The model under review builds one solid part; all positions refer to its coordinate system, in mm. Coordinates: 2 decimals unless noted, no trailing zeros. Write each loop counter-clockwise with the first axis right and the second up, starting at its lowest first coordinate (ties: lowest second). Pieces come first, ordered by that corner, then holes.
1) Add section A-A, the plane z = -0.75. State the section outline as (x, y) points, then the cut area to 3 significant figures.
2) Mouldability with a two-part tool opening along Y and no side actions: class faces 1 (the flat face through (4, 0, 0.3)), 2 (the cylindrical face through (9.84, 15.43, -0.49)), 3 (the flat face through (-6, 0, 0.2)) as released by +Y, released by -Y, zero draft, split by the parting line, or undercut.
3) For P1, Ø10, axis at x = -14, y = -10.5, coming from the +Z side; P2, Ø11.5, axis at x = 5.5, y = -1.5, coming from the -Z side, all flat-tipped, find the tip position at first contact; note any pin that passes through.
4) For line 1 (Y direction, x = 0, z = -0.5); line 2 (Z direction, x = 11, y = -12.5); line 3 (X direction, y = -6.5, z = -0.15), list the stretches that pass through material, from the lowest coordinate up.
from build123d import *

# Parameters (mm, degrees)
SKETCH1_R           = 19.5
BOSS_EXTRUDE1_DEPTH = 0.3
SKETCH1_3_R         = 18.6
SKETCH1_3_R_2       = 18.3
BOSS_EXTRUDE2_DEPTH = 1
FILLET1_R           = 10
CUT_EXTRUDE1_START  = -0.1
CUT_EXTRUDE1_DEPTH  = 0.1


# Read off the part's stored shape, not the designer's step: Cut-Extrude1
with BuildPart() as part:
    # Sketch1 → Boss-Extrude1 (new body)
    with BuildSketch(Plane.XY):
        Circle(SKETCH1_R)
    extrude(amount=BOSS_EXTRUDE1_DEPTH)

    # Sketch1<3> → Boss-Extrude2 (add)
    with BuildSketch(Plane.XY):
        Circle(SKETCH1_3_R)
        Circle(SKETCH1_3_R_2, mode=Mode.SUBTRACT)
    extrude(amount=-BOSS_EXTRUDE2_DEPTH)

    # Fillet1
    # the kernel refuses this fillet: 10 mm, written as the material it takes off along each edge
    with BuildSketch(Plane(origin=(0, 0, 0.3), x_dir=(1, 0, 0), z_dir=(0, -1, 0))) as fillet1_piece_1:
        with BuildLine():
            CenterArc((17.068950844, -10), FILLET1_R, 75.930132252, 14.069867748)
            Line((17.068950844, 0), (17.068950844, 0.2))
            Line((17.068950844, 0.2), (19.5, 0.2))
            Line((19.5, 0.2), (19.7, 0))
            ThreePointArc((19.7, 0), (19.7, -0.15), (19.548620983, -0.106))
            Line((19.548620983, -0.106), (19.5, -0.3))
        make_face()
    revolve(axis=Axis((0, 0, 0.3), (0, 0, 1)), mode=Mode.SUBTRACT)

    # Cut-Extrude1 outline → Cut-Extrude1 (cut)
    with BuildSketch(Plane.XY.offset(0.3).offset(CUT_EXTRUDE1_START)):
        with BuildLine():
            Line((1.315411857, -4.122498151), (2.014314535, -1.338720024))
            ThreePointArc((2.014314535, -1.338720024), (5.071648244, -4.189541516), (8.236226494, -1.458256637))
            Line((8.236226494, -1.458256637), (6.810434555, -1.458256637))
            ThreePointArc((6.810434555, -1.458256637), (5.012044187, -2.913884745), (3.355418791, -1.298752119))
            ThreePointArc((3.355418791, -1.298752119), (3.437417537, -0.072322093), (3.940070016, 1.049370774))
            ThreePointArc((3.940070016, 1.049370774), (5.536779658, 1.617570868), (6.80295626, 0.491014238))
            Line((6.80295626, 0.491014238), (8.236226494, 0.491014238))
            ThreePointArc((8.236226494, 0.491014238), (5.861564417, 2.797023993), (2.721821376, 1.74882811))
            Line((2.721821376, 1.74882811), (3.407587296, 4.634399496))
            Line((3.407587296, 4.634399496), (1.750846599, 4.634399496))
            Line((1.750846599, 4.634399496), (0.532539724, -1.311746329))
            Line((0.532539724, -1.311746329), (-0.832013668, 4.634399496))
            Line((-0.832013668, 4.634399496), (-2.328745068, 4.634399496))
            Line((-2.328745068, 4.634399496), (-3.653616427, -1.303011789))
            Line((-3.653616427, -1.303011789), (-4.854525711, 4.634399496))
            Line((-4.854525711, 4.634399496), (-6.247187009, 4.603807508))
            Line((-6.247187009, 4.603807508), (-4.13707531, -4.122498151))
            Line((-4.13707531, -4.122498151), (-2.868545937, -4.122498151))
            Line((-2.868545937, -4.122498151), (-1.610862761, 1.75217424))
            Line((-1.610862761, 1.75217424), (-0.291169429, -4.122498151))
            Line((-0.291169429, -4.122498151), (1.315411857, -4.122498151))
        make_face()
        with BuildLine():
            Line((-6.937538905, -2.602863273), (-6.637674337, -2.602863273))
            ThreePointArc((-6.637674337, -2.602863273), (-6.120559929, -2.872899906), (-5.547687427, -2.983100592))
            Line((-5.547687427, -2.983100592), (-5.062190332, -2.983100592))
            Line((-5.062190332, -2.983100592), (-4.643328191, -4.157083976))
            Line((-4.643328191, -4.157083976), (-4.338702943, -4.157083976))
            Line((-4.338702943, -4.157083976), (-6.406435712, 4.616022013))
            Line((-6.406435712, 4.616022013), (-6.794480732, 4.524563708))
            Line((-6.794480732, 4.524563708), (-6.497707451, 2.844057166))
            ThreePointArc((-6.497707451, 2.844057166), (-6.543403682, 2.764133189), (-6.634976133, 2.773644958))
            ThreePointArc((-6.634976133, 2.773644958), (-6.812471334, 2.860826812), (-7.00818234, 2.832499724))
            ThreePointArc((-7.00818234, 2.832499724), (-7.232944109, 2.4137084), (-6.990239601, 2.005053843))
            ThreePointArc((-6.990239601, 2.005053843), (-6.671904577, 2.052546685), (-6.464198285, 2.298414239))
            Line((-6.464198285, 2.298414239), (-6.400014039, 2.298414239))
            Line((-6.400014039, 2.298414239), (-6.400014039, 2.081303951))
            ThreePointArc((-6.400014039, 2.081303951), (-6.496019237, 1.38621962), (-6.377516068, 0.694615526))
            Line((-6.377516068, 0.694615526), (-7.103342547, -0.4012317))
            ThreePointArc((-7.103342547, -0.4012317), (-7.155024922, -0.494114517), (-7.158413077, -0.600353898))
            ThreePointArc((-7.158413077, -0.600353898), (-7.020194568, -0.758643223), (-6.815959597, -0.808119916))
            ThreePointArc((-6.815959597, -0.808119916), (-6.877232982, -0.649384136), (-6.826115409, -0.487092826))
            Line((-6.826115409, -0.487092826), (-6.666005475, -0.342790453))
            ThreePointArc((-6.666005475, -0.342790453), (-6.364107135, -0.25949819), (-6.071279663, -0.37054899))
            ThreePointArc((-6.071279663, -0.37054899), (-5.738084346, -0.734492432), (-5.554908519, -1.192663322))
            Line((-5.554908519, -1.192663322), (-5.636587076, -1.257125772))
            Line((-5.636587076, -1.257125772), (-5.52013275, -1.803631749))
            ThreePointArc((-5.52013275, -1.803631749), (-5.60809608, -2.112628848), (-5.913172695, -2.213351306))
            ThreePointArc((-5.913172695, -2.213351306), (-6.401983276, -1.969270784), (-6.837380228, -1.639209304))
            ThreePointArc((-6.837380228, -1.639209304), (-7.277778062, -2.310157247), (-7.410559234, -3.101668811))
            ThreePointArc((-7.410559234, -3.101668811), (-7.217893073, -3.146992956), (-7.172568928, -2.954326795))
            ThreePointArc((-7.172568928, -2.954326795), (-7.105944543, -2.74456355), (-6.937538905, -2.602863273))
        make_face()
    extrude(amount=CUT_EXTRUDE1_DEPTH, mode=Mode.SUBTRACT)


solid = part.part
Geometry results:
1. outline: circle Ø37.2 at (0, 0); hole circle Ø36.6 at (0, 0)
1. area: 34.8 mm2
2. face 1: zero draft
2. face 2: undercut
2. face 3: undercut
3. P1: stops at z = 0.3
3. P2: stops at z = 0
4. line 1: y = -18.6 to -18.3, 18.3 to 18.6
4. line 2: z = 0 to 0.3
4. line 3: x = -17.43 to -17.11, 17.11 to 17.43
